```python
from build123d import *

# Parameters (mm, degrees)
ESQUISSE1_W                    = 42
ESQUISSE1_H                    = 52
BOSS_EXTRU_1_DEPTH             = 3.3
ESQUISSE3_W                    = 3.3
ESQUISSE3_H                    = 8
BOSS_EXTRU_2_DEPTH             = 3.3
R_P_TITION_LIN_AIRE1_COUNT     = 3
R_P_TITION_LIN_AIRE1_PITCH     = 16
R_P_TITION_LIN_AIRE1_COL_COUNT = 2
R_P_TITION_LIN_AIRE1_COL_PITCH = 16
SYM_TRIE1_COPY_1_SKETCH_W      = 3.3
SYM_TRIE1_COPY_1_SKETCH_H      = 8
SYM_TRIE1_COPY_1_DEPTH         = 3.3
SYM_TRIE1_COPY_2_SKETCH_W      = 3.3
SYM_TRIE1_COPY_2_SKETCH_H      = 8
SYM_TRIE1_COPY_2_DEPTH         = 3.3
SYM_TRIE1_COPY_3_SKETCH_W      = 3.3
SYM_TRIE1_COPY_3_SKETCH_H      = 8
SYM_TRIE1_COPY_3_DEPTH         = 3.3
ESQUISSE4_W                    = 8
ESQUISSE4_H                    = 3.3
BOSS_EXTRU_3_DEPTH             = 3.3
R_P_TITION_LIN_AIRE2_COUNT     = 3
R_P_TITION_LIN_AIRE2_PITCH     = 16
R_P_TITION_LIN_AIRE2_COL_COUNT = 2
R_P_TITION_LIN_AIRE2_COL_PITCH = 16
ESQUISSE5_W                    = 3.7
ESQUISSE5_H                    = 3.3
ENL_V_MAT_EXTRU_1_DEPTH        = 41.661775662
SYM_TRIE2_START                = -29.3
SYM_TRIE2_OUTLINE_W            = 4.3
SYM_TRIE2_OUTLINE_H            = 3.3
SYM_TRIE2_OUTLINE_W_2          = 8
SYM_TRIE2_DEPTH                = 3.3


# Read off the part's stored shape, not the designer's step: Symétrie2
with BuildPart() as part:
    # Esquisse1 → Boss.-Extru.1 (new body)
    with BuildSketch(Plane.XY):
        Rectangle(ESQUISSE1_W, ESQUISSE1_H)
    extrude(amount=BOSS_EXTRU_1_DEPTH)

    # Esquisse3 → Boss.-Extru.2 (add)
    with BuildSketch(Plane.XY.offset(3.3)):
        with Locations((22.65, -8)):
            Rectangle(ESQUISSE3_W, ESQUISSE3_H)
    boss_extru_2 = extrude(amount=-BOSS_EXTRU_2_DEPTH)

    # Répétition linéaire1: Boss.-Extru.2 ×3
    with Locations(*[(0, i * R_P_TITION_LIN_AIRE1_PITCH, 0) for i in range(1, R_P_TITION_LIN_AIRE1_COUNT)]):
        add(boss_extru_2)

    # Répétition linéaire1 col: Boss.-Extru.2 ×2
    with Locations(*[(0, -i * R_P_TITION_LIN_AIRE1_COL_PITCH, 0) for i in range(1, R_P_TITION_LIN_AIRE1_COL_COUNT)]):
        add(boss_extru_2)

    # Symétrie1: Boss.-Extru.2 across plane
    add(boss_extru_2.mirror(Plane(origin=(0, 0, 0), x_dir=(0, 0, 1), z_dir=(1, 0, 0))))

    # Symétrie1 copy 1 sketch → Symétrie1 copy 1 (add)
    with BuildSketch(Plane(origin=(0, 16, 3.3), x_dir=(-1, 0, 0), z_dir=(0, 0, 1))):
        with Locations((22.65, 8)):
            Rectangle(SYM_TRIE1_COPY_1_SKETCH_W, SYM_TRIE1_COPY_1_SKETCH_H)
    extrude(amount=-SYM_TRIE1_COPY_1_DEPTH)

    # Symétrie1 copy 2 sketch → Symétrie1 copy 2 (add)
    with BuildSketch(Plane(origin=(0, 32, 3.3), x_dir=(-1, 0, 0), z_dir=(0, 0, 1))):
        with Locations((22.65, 8)):
            Rectangle(SYM_TRIE1_COPY_2_SKETCH_W, SYM_TRIE1_COPY_2_SKETCH_H)
    extrude(amount=-SYM_TRIE1_COPY_2_DEPTH)

    # Symétrie1 copy 3 sketch → Symétrie1 copy 3 (add)
    with BuildSketch(Plane(origin=(0, -16, 3.3), x_dir=(-1, 0, 0), z_dir=(0, 0, 1))):
        with Locations((22.65, 8)):
            Rectangle(SYM_TRIE1_COPY_3_SKETCH_W, SYM_TRIE1_COPY_3_SKETCH_H)
    extrude(amount=-SYM_TRIE1_COPY_3_DEPTH)

    # Esquisse4 → Boss.-Extru.3 (add)
    with BuildSketch(Plane.XY.offset(3.3)):
        with Locations((-8, 27.65)):
            Rectangle(ESQUISSE4_W, ESQUISSE4_H)
    boss_extru_3 = extrude(amount=-BOSS_EXTRU_3_DEPTH)

    # Répétition linéaire2: Boss.-Extru.3 ×3
    with Locations(*[(i * R_P_TITION_LIN_AIRE2_PITCH, 0, 0) for i in range(1, R_P_TITION_LIN_AIRE2_COUNT)]):
        add(boss_extru_3)

    # Répétition linéaire2 col: Boss.-Extru.3 ×2
    with Locations(*[(-i * R_P_TITION_LIN_AIRE2_COL_PITCH, 0, 0) for i in range(1, R_P_TITION_LIN_AIRE2_COL_COUNT)]):
        add(boss_extru_3)

    # Esquisse5 → Enlèv. mat.-Extru.1 (cut, symmetric)
    with BuildSketch(Plane.XY.offset(3.3)):
        with Locations((-26.15, 27.65)):
            Rectangle(ESQUISSE5_W, ESQUISSE5_H)
        with Locations((26.15, 27.65)):
            Rectangle(ESQUISSE5_W, ESQUISSE5_H)
    extrude(amount=ENL_V_MAT_EXTRU_1_DEPTH, both=True, mode=Mode.SUBTRACT)

    # Symétrie2 outline → Symétrie2 (add)
    with BuildSketch(Plane(origin=(0, 0, 0), x_dir=(1, 0, 0), z_dir=(0, 1, 0)).offset(SYM_TRIE2_START)):
        with Locations((22.15, -1.65)):
            Rectangle(SYM_TRIE2_OUTLINE_W, SYM_TRIE2_OUTLINE_H)
        with Locations((8, -1.65)):
            Rectangle(SYM_TRIE2_OUTLINE_W_2, SYM_TRIE2_OUTLINE_H)
        with Locations((-8, -1.65)):
            Rectangle(SYM_TRIE2_OUTLINE_W_2, SYM_TRIE2_OUTLINE_H)
        with Locations((-22.15, -1.65)):
            Rectangle(SYM_TRIE2_OUTLINE_W, SYM_TRIE2_OUTLINE_H)
    extrude(amount=SYM_TRIE2_DEPTH)


solid = part.part
```
Check sheet for the modelled part. Datum: model origin and axes. Units: mm. A direction names the side the tool comes from. Give positions to 0.01 mm unless a question says otherwise; leave off trailing zeros. Loops run counter-clockwise (first coordinate to the right, second up) from the corner with the lowest first, then second, coordinate; pieces in that order, holes last. Notation, with made-up numbers: M -18.5,72.25 L 24.5,72.25 A25 cw 24.5,109.25 Z; hole C 19.5,20 d11. An arc over 180 degrees is marked long. Answer in a Markdown table with one row per item.
1) Cross-section at B-B (y = 16). Enter the section's corners in (x, z), plus the area to 3 significant figures.
Solutions:
| item | result |
|---|---|
| outline | M -21,0 L 21,0 L 21,3.3 L -21,3.3 Z |
| area | 139 mm^2 |
2) Tool access check on faces 5 (the face through (21, 16, 2)), 6 (the face through (20, 28, 2)), 7 (the face through (-4, -28, 2)). Record the directions out of +Z, -Z, +X, -X, +Y, -Y that give a thin tool (end or side, any length) a straight path to the whole face; none if there is none.
Solutions:
| item | result |
|---|---|
| face 5 | +Z, -Z, +X |
| face 6 | +Z, -Z, +Y |
| face 7 | +Z, -Z, -Y |
3) Mould release check, pull along Y, two halves, no side actions. Record for faces 1 (the face through (-21, 16, 2)), 2 (the face through (4, -28, 2)), 3 (the face through (-21, 0, 2)), 4 (the face through (0, 26, 2)): released by +Y, released by -Y, zero draft, split by the parting line, or undercut.
Solutions:
| item | result |
|---|---|
| face 1 | undercut |
| face 2 | zero draft |
| face 3 | undercut |
| face 4 | released by +Y |
4) Depth check by flat-ended pin: pin 1 (1 mm diameter, centred on x = -15.5, z = 1.5, fed in from -Y); pin 2 (1 mm diameter, centred on y = 15, z = 1.5, fed in from +X). Enter the tip coordinate at first touch or a pass-through.
Solutions:
| item | result |
|---|---|
| pin 1 | stops at y = -26 |
| pin 2 | stops at x = 21 |
5) Cross-section at A-A (x = 0.5). Enter the section's corners in (y, z), plus the area to 3 significant figures.
Solutions:
| item | result |
|---|---|
| outline | M -26,0 L 26,0 L 26,3.3 L -26,3.3 Z |
| area | 172 mm^2 |
6) Thickness scan on line 1 (Y direction, x = 21.5, z = 3); line 2 (X direction, y = 27, z = 1.35); line 3 (Y direction, x = -3, z = 0.3). Record the ranges inside material, lowest first.
Solutions:
| item | result |
|---|---|
| line 1 | y = -29.3 to -20, -12 to -4, 4 to 12, 20 to 29.3 |
| line 2 | x = -24.3 to -20, -12 to -4, 4 to 12, 20 to 24.3 |
| line 3 | y = -26 to 26 |
